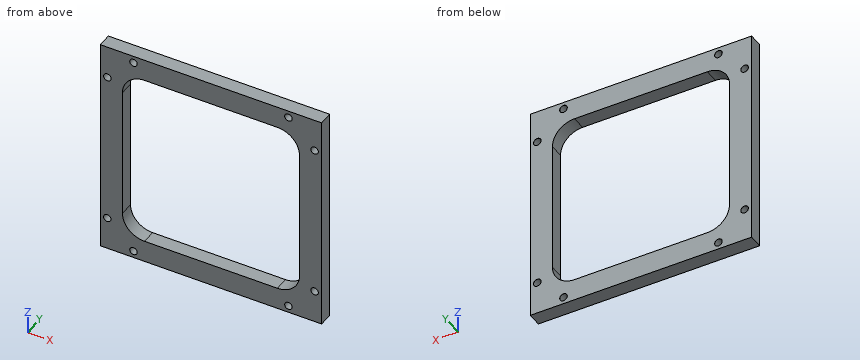
from build123d import *

# Parameters (mm, degrees)
SKETCH1_W                      = 100
SKETCH1_H                      = 100
BOSS_EXTRUDE3_DEPTH            = 6.35
M3_CLEARANCE_HOLE1_D           = 3.4
M3_CLEARANCE_HOLE1_CSINK_D     = 3.45
M3_CLEARANCE_HOLE1_CSINK_ANGLE = 90
CUT_EXTRUDE1_DEPTH             = 10


with BuildPart() as part:
    # Sketch1 → Boss-Extrude3 (new body)
    with BuildSketch(Plane(origin=(0, 0, 0), x_dir=(1, 0, 0), z_dir=(0, 1, 0))):
        Rectangle(SKETCH1_W, SKETCH1_H)
    extrude(amount=BOSS_EXTRUDE3_DEPTH)

    # M3 Clearance Hole1 (through all)
    with Locations(Plane(origin=(0, 6.35, 0), x_dir=(1, 0, 0), z_dir=(0, 1, 0))):
        with Locations((-46.825, 35), (-35, 46.825), (35, 46.825), (46.825, 35), (46.825, -35), (35, -46.825), (-35, -46.825), (-46.825, -35)):
            CounterSinkHole(M3_CLEARANCE_HOLE1_D / 2, M3_CLEARANCE_HOLE1_CSINK_D / 2, counter_sink_angle=M3_CLEARANCE_HOLE1_CSINK_ANGLE)

    # Sketch19 → Cut-Extrude1 (cut)
    with BuildSketch(Plane(origin=(0, 6.35, 0), x_dir=(1, 0, 0), z_dir=(0, 1, 0))):
        with BuildLine():
            Line((-30, -40), (30, -40))
            ThreePointArc((30, -40), (37.071067812, -37.071067812), (40, -30))
            Line((40, -30), (40, 30))
            ThreePointArc((40, 30), (37.071067812, 37.071067812), (30, 40))
            Line((30, 40), (-30, 40))
            ThreePointArc((-30, 40), (-37.071067812, 37.071067812), (-40, 30))
            Line((-40, 30), (-40, -30))
            ThreePointArc((-40, -30), (-37.071067812, -37.071067812), (-30, -40))
        make_face()
    extrude(amount=-CUT_EXTRUDE1_DEPTH, mode=Mode.SUBTRACT)


solid = part.part
Geometry check sheet. Reference: the model listing, model coordinates, mm. Give positions to 0.01 mm unless a question says otherwise; leave off trailing zeros. Loops run counter-clockwise (first coordinate to the right, second up) from the corner with the lowest first, then second, coordinate; pieces in that order, holes last.
(1) Thickness scan on L1, parallel to X at y = 1.5, z = -35 (3 decimals); L2, parallel to X at y = 4.5, z = 22. Record the ranges inside material, lowest first.
From the geometry:
L1: x = -50 to -48.525, -45.125 to -38.66, 38.66 to 45.125, 48.525 to 50
L2: x = -50 to -40, 40 to 50
(2) Section check C-C on y = 3. Count the separate pieces of the cut face and the enclosed holes in it, then the cut area to 3 significant figures.
From the geometry:
separate pieces: 1
enclosed holes: 9
area: 3,610 mm2
(3) Section check D-D on z = -35. Record the cut outline in (x, y) (3 decimals).
From the geometry:
outline: (-50, 0) - (-48.525, 0) - (-48.525, 6.325) - (-48.55, 6.35) - (-50, 6.35) - close; (-45.125, 0) - (-38.66, 0) - (-38.66, 6.35) - (-45.1, 6.35) - (-45.125, 6.325) - close; (38.66, 0) - (45.125, 0) - (45.125, 6.325) - (45.1, 6.35) - (38.66, 6.35) - close; (48.525, 0) - (50, 0) - (50, 6.35) - (48.55, 6.35) - (48.525, 6.325) - close
(4) Section check A-A on z = 38. Record the cut outline in (x, y).
From the geometry:
outline: (-50, 0) - (-36, 0) - (-36, 6.35) - (-50, 6.35) - close; (36, 0) - (50, 0) - (50, 6.35) - (36, 6.35) - close
(5) Section check B-B on x = 26.5. Record the cut outline in (y, z), then the cut area to 3 significant figures.
From the geometry:
outline: (0, -50) - (6.35, -50) - (6.35, -40) - (0, -40) - close; (0, 40) - (6.35, 40) - (6.35, 50) - (0, 50) - close
area: 127 mm2
